Input: part model. Units: mm. Frame: model coordinates. A direction names the side the tool comes from. Coordinates: 2 decimals unless noted, no trailing zeros. Loops run counter-clockwise (first coordinate to the right, second up) from the corner with the lowest first, then second, coordinate; pieces in that order, holes last.
```python
from build123d import *

# Parameters (mm, degrees)
SKETCH1_W           = 304.8
SKETCH1_H           = 304.8
BOSS_EXTRUDE1_DEPTH = 38.1
CUT_EXTRUDE1_DEPTH  = 305.8
LPATTERN1_COUNT     = 12
LPATTERN1_PITCH     = 25.4


with BuildPart() as part:
    # Sketch1 → Boss-Extrude1 (new body)
    with BuildSketch(Plane(origin=(0, 0, 0), x_dir=(1, 0, 0), z_dir=(0, 1, 0))):
        with Locations((152.4, -152.4)):
            Rectangle(SKETCH1_W, SKETCH1_H)
    extrude(amount=BOSS_EXTRUDE1_DEPTH)

    # Sketch2 → Cut-Extrude1 (cut, through all)
    with BuildSketch(Plane.XY.offset(304.8)):
        Polygon((0, 38.1), (12.7, 19.05), (25.4, 38.1), align=None)
    cut_extrude1 = extrude(amount=-CUT_EXTRUDE1_DEPTH, mode=Mode.SUBTRACT)

    # LPattern1: Cut-Extrude1 ×12
    with Locations(*[(i * LPATTERN1_PITCH, 0, 0) for i in range(1, LPATTERN1_COUNT)]):
        add(cut_extrude1, mode=Mode.SUBTRACT)


solid = part.part
```
Item 1: Mould query, pull axis X, two halves, no side actions, for faces 3 (the face through (150, 15, 0)), 4 (the face through (158.66, 28.71, 154.53)), 5 (the face through (69.76, 28.44, 154.53)). Classes: +X half, -X half, draft (parallel to the pull), parting line (faces both ways), or undercut.
Result:
face 3: draft
face 4: undercut
face 5: undercut
Item 2: Section query D-D (x = 58). Output: boundary loops of the cut face in (y, z).
Result:
outline: (0, 0) - (27.3, 0) - (27.3, 304.8) - (0, 304.8) - close
Item 3: Section query A-A (z = 247.5). Output: boundary loops of the cut face in (x, y), then the cut area to 3 significant figures.
Result:
outline: (0, 0) - (304.8, 0) - (304.8, 38.1) - (292.1, 19.05) - (279.4, 38.1) - (266.7, 19.05) - (254, 38.1) - (241.3, 19.05) - (228.6, 38.1) - (215.9, 19.05) - (203.2, 38.1) - (190.5, 19.05) - (177.8, 38.1) - (165.1, 19.05) - (152.4, 38.1) - (139.7, 19.05) - (127, 38.1) - (114.3, 19.05) - (101.6, 38.1) - (88.9, 19.05) - (76.2, 38.1) - (63.5, 19.05) - (50.8, 38.1) - (38.1, 19.05) - (25.4, 38.1) - (12.7, 19.05) - (0, 38.1) - close
area: 8,710 mm2
Item 4: Section query B-B (y = 31.5). Count the separate pieces of the cut face and the enclosed holes in it, then the cut area to 3 significant figures.
Result:
separate pieces: 13
enclosed holes: 0
area: 32,200 mm2
Item 5: Line query: L1, parallel to Y at x = 107, z = 71; L2, parallel to Y at x = 221, z = 237.5. Output: solid intervals per line, ascending.
Result:
L1: y = 0 to 30
L2: y = 0 to 26.7
Item 6: Section query C-C (x = 118). Output: boundary loops of the cut face in (y, z).
Result:
outline: (0, 0) - (24.6, 0) - (24.6, 304.8) - (0, 304.8) - close
Item 7: Reachability of faces 1 (the face through (150, 0, 150)), 2 (the face through (6.26, 28.71, 154.53)) from +Z, -Z, +X, -X, +Y, -Y: full face, straight path, thin tool, end or side. Return the list, or none.
Result:
face 1: +Z, -Z, +X, -X, -Y
face 2: +Z, -Z, +Y
